from build123d import *

# Parameters (mm, degrees)
BOSS_EXTRUDE1_DEPTH = 12.7


with BuildPart() as part:
    # Sketch2 → Boss-Extrude1 (new body)
    with BuildSketch(Plane(origin=(0, 0, 0), x_dir=(1, 0, 0), z_dir=(0, 1, 0))):
        Polygon((-23.625933555, 44.491909321), (23.625933555, 44.491909321), (38.1, 52.84851548), (50.8, 45.516167061), (50.8, 30.851470224), (44.45, 27.185296014), (44.45, -27.101477372), (50.8, -30.767651581), (50.8, -45.432348419), (38.1, -52.764696837), (23.625933555, -44.408090679), (-23.625933555, -44.408090679), (-38.1, -52.764696837), (-50.8, -45.432348419), (-50.8, -30.767651581), (-44.45, -27.101477372), (-44.45, 27.185296014), (-50.8, 30.851470224), (-50.8, 45.516167061), (-38.1, 52.84851548), align=None)
        Polygon((-38.1, 45.516167061), (-44.45, 41.849992852), (-44.45, 34.517644433), (-38.1, 30.851470224), (-31.75, 34.517644433), (-31.75, 41.849992852), align=None, mode=Mode.SUBTRACT)
        Polygon((38.1, 45.516167061), (31.75, 41.849992852), (31.75, 34.517644433), (38.1, 30.851470224), (44.45, 34.517644433), (44.45, 41.849992852), align=None, mode=Mode.SUBTRACT)
        Polygon((-38.1, -30.767651581), (-44.45, -34.433825791), (-44.45, -41.766174209), (-38.1, -45.432348419), (-31.75, -41.766174209), (-31.75, -34.433825791), align=None, mode=Mode.SUBTRACT)
        Polygon((38.1, -30.767651581), (31.75, -34.433825791), (31.75, -41.766174209), (38.1, -45.432348419), (44.45, -41.766174209), (44.45, -34.433825791), align=None, mode=Mode.SUBTRACT)
        Polygon((0, 23.547094971), (-22.394618112, 7.276452514), (-13.840635159, -19.05), (13.840635159, -19.05), (22.394618112, 7.276452514), align=None, mode=Mode.SUBTRACT)
    extrude(amount=BOSS_EXTRUDE1_DEPTH)


solid = part.part
Verification items for the finished model (mm, model axes). A direction names the side the tool comes from. Give positions to 0.01 mm unless a question says otherwise; leave off trailing zeros. Write each loop counter-clockwise with the first axis right and the second up, starting at its lowest first coordinate (ties: lowest second). Pieces come first, ordered by that corner, then holes. Notation, with made-up numbers: M 66.25,-18.5 L 83.25,-18.5 A17 cw 83.25,-5.5 Z; hole C -15.75,42.25 d9. An arc over 180 degrees is marked long. Put each result on its own line as item: value. Start each with the question number.
1. Scan lines: line 1 along X through (y, z) = (11.25, -40.5); line 2 along Z through (x, y) = (-42.5, 10); line 3 along X through (y, z) = (6.75, 45). Record each from-to range of solid material in increasing order. Write a range as [from, to].
2. Go/stop test with flat-tipped pins: pin 1 Ø3 at (x, y) = (2, 4) entering from -Z; pin 2 Ø6.5 at (y, z) = (3, -10) entering from -X; pin 3 Ø1 at (y, z) = (11, -20) entering from +X. Record where each tip stops, or that it passes through.
3. Section check C-C (z = -12.5). Record the cut outline in (x, y), and give its area (3 significant figures).
4. Section check B-B (x = -19.5). Record the cut outline in (y, z).
5. Set-up check for faces 4 (the face through (34.97, 6.26, -43.71)), 5 (the face through (50.8, 6, 38)), 6 (the face through (44.45, 6, 0)), 7 (the face through (30.76, 6.26, -48.61)), 8 (the face through (-47.67, 6.26, 28.96)): record each of +Z, -Z, +X, -X, +Y, -Y from which the full face is reachable in a straight line by a thin tool's end or side.
6. Section check D-D (x = 36.5). Record the cut outline in (y, z), and give its area (3 significant figures).
7. Section check A-A (z = 37). Record the cut outline in (x, y).
8. Draft check along X on faces 1 (the face through (47.669, 6.261, -29.044)), 2 (the face through (34.881, 6.261, 43.574)), 3 (the face through (-47.581, 6.261, -28.993)). Enter one of: +X half, -X half, draft (parallel to the pull), parting line (faces both ways), or undercut.
Answer list:
1. line 1: [-50.8, -44.45], [-31.75, 31.75], [44.45, 50.8]
1. line 2: [-50.31, -42.98], [-33.39, 33.31], [42.89, 50.22]
1. line 3: [-50.8, -38.85], [-37.35, -24.65], [24.65, 37.35], [38.85, 50.8]
2. pin 1: z = -44.49
2. pin 2: x = -44.45
2. pin 3: x = 44.45
3. outline: M -44.45,0 L -15.21,0 L -15.21,12.7 L -44.45,12.7 Z; M 15.21,0 L 44.45,0 L 44.45,12.7 L 15.21,12.7 Z
3. area: 743 mm2
4. outline: M 0,-44.49 L 12.7,-44.49 L 12.7,-9.38 L 0,-9.38 Z; M 0,1.63 L 12.7,1.63 L 12.7,44.41 L 0,44.41 Z
5. face 4: +Y, -Y
5. face 5: +Z, -Z, +X, +Y, -Y
5. face 6: +X, +Y, -Y
5. face 7: -Z, +Y, -Y
5. face 8: -X, +Y, -Y
6. outline: M 0,-51.92 L 12.7,-51.92 L 12.7,-44.59 L 0,-44.59 Z; M 0,-31.78 L 12.7,-31.78 L 12.7,31.69 L 0,31.69 Z; M 0,44.51 L 12.7,44.51 L 12.7,51.84 L 0,51.84 Z
6. area: 992 mm2
7. outline: M -50.8,0 L -44.45,0 L -44.45,12.7 L -50.8,12.7 Z; M -31.75,0 L 31.75,0 L 31.75,12.7 L -31.75,12.7 Z; M 44.45,0 L 50.8,0 L 50.8,12.7 L 44.45,12.7 Z
8. face 1: +X half
8. face 2: undercut
8. face 3: -X half
